Check sheet for the modelled part. Datum: model origin and axes. Units: mm. Coordinates: 2 decimals unless noted, no trailing zeros. Write each loop counter-clockwise with the first axis right and the second up, starting at its lowest first coordinate (ties: lowest second). Pieces come first, ordered by that corner, then holes. Notation, with made-up numbers: (3, 84) - (54, 84) arc R11 cw to (54, 105) - close; hole circle Ø7 at (-11.75, 74.25). An arc over 180 degrees is marked (long way). Write each question's results on one line, items separated by ' | '.
from build123d import *

# Parameters (mm, degrees)
F0_W      = 6.5
F0_H      = 6.5
F1_DEPTH  = 6.5
F2_R      = 1
F3_DEPTH  = 25
F4_W      = 0.5
F4_H      = 6.5
F5_DEPTH  = 0.2
F6_W      = 6.3
F6_H      = 0.5
F7_DEPTH  = 0.2
F8_W      = 0.5
F8_H      = 6.3
F9_DEPTH  = 0.2
F10_W     = 6.1
F10_H     = 0.5
F11_DEPTH = 0.2


with BuildPart() as f1:
    # F0 (on Front) → F1 (new body)
    with BuildSketch(Plane.XZ):
        with Locations((3.25, -3.25)):
            Rectangle(F0_W, F0_H)
    extrude(amount=F1_DEPTH)

    # F2 (on face) → F3 (cut)
    with BuildSketch(Plane.XZ.offset(6.5)):
        with Locations((3.25, -3.25)):
            Circle(F2_R)
    extrude(amount=-F3_DEPTH, mode=Mode.SUBTRACT)

    # F4 (on face) → F5 (cut)
    with BuildSketch(Plane.YZ.offset(6.5)):
        with Locations((-5.75, -3.25)):
            Rectangle(F4_W, F4_H)
        with Locations((-4.95, -3.25)):
            Rectangle(F4_W, F4_H)
        Polygon((-3.1, 0), (-3.1, -6.5), (-2.6, -6.5), (-2.6, -2.0569080953), (-1, -0.6072367541), (-1, -6.5), (-0.5, -6.5), (-0.5, 0), (-1, 0), (-1, -0.1072367541), (-2.6, -1.5569080953), (-2.6, 0), align=None)
    extrude(amount=-F5_DEPTH, mode=Mode.SUBTRACT)

    # F6 (on face) → F7 (cut)
    with BuildSketch(Plane.XY):
        with Locations((3.15, -5.75)):
            Rectangle(F6_W, F6_H)
        with Locations((3.15, -4.95)):
            Rectangle(F6_W, F6_H)
        Polygon((0, -2.6), (0, -3.1), (6.3, -3.1), (6.3, -2.6), (2.0569080953, -2.6), (0.6072367541, -1), (6.3, -1), (6.3, -0.5), (0, -0.5), (0, -1), (0.1072367541, -1), (1.5569080953, -2.6), align=None)
    extrude(amount=-F7_DEPTH, mode=Mode.SUBTRACT)

    # F8 (on face) → F9 (cut)
    with BuildSketch(Plane(origin=(0, 0, 0), x_dir=(0, -1, 0), z_dir=(-1, 0, 0))):
        with Locations((5.75, -3.35)):
            Rectangle(F8_W, F8_H)
        with Locations((4.95, -3.35)):
            Rectangle(F8_W, F8_H)
        Polygon((2.6, -6.5), (3.1, -6.5), (3.1, -0.2), (2.6, -0.2), (2.6, -4.3532891255), (1, -5.8029604666), (1, -0.2), (0.5, -0.2), (0.5, -6.5), (1, -6.5), (1, -6.3029604666), (2.6, -4.8532891255), align=None)
    extrude(amount=-F9_DEPTH, mode=Mode.SUBTRACT)

    # F10 (on face) → F11 (cut)
    with BuildSketch(Plane(origin=(0, 0, -6.5), x_dir=(1, 0, 0), z_dir=(0, 0, -1))):
        with Locations((3.25, 5.75)):
            Rectangle(F10_W, F10_H)
        with Locations((3.25, 4.95)):
            Rectangle(F10_W, F10_H)
        Polygon((6.3, 3.1), (0.2, 3.1), (0.2, 2.6), (4.4430919047, 2.6), (5.8927632459, 1), (0.2, 1), (0.2, 0.5), (6.3, 0.5), (6.3, 1), (6.3927632459, 1), (4.9430919047, 2.6), (6.3, 2.6), align=None)
    extrude(amount=-F11_DEPTH, mode=Mode.SUBTRACT)


solid = f1.part
1. Sectioned sample at A-A (y = -4.25). Record the cut outline in (x, z).
Values follow:
outline: (0, -6.5) - (6.5, -6.5) - (6.5, 0) - (0, 0) - close; hole circle Ø2 at (3.25, -3.25)
2. Material ranges on L1, parallel to Z at x = 3.25, y = -2.25; L2, parallel to X at y = -0.75, z = -6; L3, parallel to Z at x = 1.25, y = -1.75, recorded low to high. Write a range as [from, to].
Values follow:
L1: z = [-6.5, -4.25], [-2.25, 0] | L2: x = [0.2, 6.3] | L3: z = [-6.5, -0.2]
3. Sectioned sample at B-B (y = -1.25). Record the cut outline in (x, z), then the cut area to 3 significant figures.
Values follow:
outline: (0, -6.5) - (5.67, -6.5) - (5.67, -6.3) - (6.17, -6.3) - (6.17, -6.5) - (6.5, -6.5) - (6.5, -0.83) - (6.3, -0.83) - (6.3, -0.33) - (6.5, -0.33) - (6.5, 0) - (0.83, 0) - (0.83, -0.2) - (0.33, -0.2) - (0.33, 0) - (0, 0) - (0, -5.58) - (0.2, -5.58) - (0.2, -6.08) - (0, -6.08) - close; hole circle Ø2 at (3.25, -3.25) | area: 38.7 mm^2
